```python
from build123d import *

# Parameters (mm, degrees)
SKETCH1_W           = 19.05
SKETCH1_H           = 22.225
BASE_FLANGE1_DEPTH  = 3.175
EDGE_FLANGE1_DEPTH  = 22.225
EDGE_FLANGE2_DEPTH  = 22.225
CUT_EXTRUDE1_DEPTH  = 42.119074421
SKETCH13_W          = 9.525
SKETCH13_H          = 3.175
BOSS_EXTRUDE1_DEPTH = 3.175
CUT_EXTRUDE2_DEPTH  = 35.761376285


# Sheet-metal steps are written as plain solids
with BuildPart() as part:
    # Sketch1 → Base-Flange1 (new body)
    with BuildSketch(Plane.XY):
        Rectangle(SKETCH1_W, SKETCH1_H)
    extrude(amount=-BASE_FLANGE1_DEPTH)

    # Edge-Flange1 section (across the edge) → Edge-Flange1 (add)
    with BuildSketch(Plane(origin=(10.525, 11.1125, -3.175), x_dir=(-1, 0, 0), z_dir=(0, -1, 0))):
        with BuildLine():
            Line((-3.175, 1), (-3.175, 25.4))
            Line((-3.175, 25.4), (0, 25.4))
            Line((0, 25.4), (0, 1))
            ThreePointArc((0, 1), (0.292893219, 0.292893219), (1, 0))
            Line((1, 0), (1, -3.175))
            ThreePointArc((1, -3.175), (-1.952170811, -1.952170811), (-3.175, 1))
        make_face()
    extrude(amount=EDGE_FLANGE1_DEPTH)

    # Edge-Flange2 section (across the edge) → Edge-Flange2 (add)
    with BuildSketch(Plane(origin=(-10.525, -11.1125, -3.175), x_dir=(1, 0, 0), z_dir=(0, 1, 0))):
        with BuildLine():
            Line((-3.175, 1), (-3.175, 25.4))
            Line((-3.175, 25.4), (0, 25.4))
            Line((0, 25.4), (0, 1))
            ThreePointArc((0, 1), (0.292893219, 0.292893219), (1, 0))
            Line((1, 0), (1, -3.175))
            ThreePointArc((1, -3.175), (-1.952170811, -1.952170811), (-3.175, 1))
        make_face()
    extrude(amount=EDGE_FLANGE2_DEPTH)

    # Sketch12 → Cut-Extrude1 (cut, through all)
    with BuildSketch(Plane(origin=(13.7, 0, 0), x_dir=(0, 0, -1), z_dir=(1, 0, 0))):
        Polygon((28.575, 11.1125), (7.35, 11.1125), (28.575, -7.9375), align=None)
    extrude(amount=-CUT_EXTRUDE1_DEPTH, mode=Mode.SUBTRACT)

    # Sketch13 → Boss-Extrude1 (add)
    with BuildSketch(Plane.XZ.offset(11.1125)):
        with Locations((0, -1.5875)):
            Rectangle(SKETCH13_W, SKETCH13_H)
    extrude(amount=BOSS_EXTRUDE1_DEPTH)

    # Sketch14 → Cut-Extrude2 (cut, through all)
    with BuildSketch(Plane.XY):
        with BuildLine():
            ThreePointArc((-3, 1.5875), (0, -1.4125), (3, 1.5875))
            Line((3, 1.5875), (-3, 1.5875))
        make_face()
        with BuildLine():
            Line((-3, 1.5875), (3, 1.5875))
            ThreePointArc((3, 1.5875), (0, 4.5875), (-3, 1.5875))
        make_face()
    extrude(amount=-CUT_EXTRUDE2_DEPTH, mode=Mode.SUBTRACT)


solid = part.part
```
Input: part model. Units: mm. Frame: model coordinates. A direction names the side the tool comes from. Give positions to 0.01 mm unless a question says otherwise; leave off trailing zeros. Loops run counter-clockwise (first coordinate to the right, second up) from the corner with the lowest first, then second, coordinate; pieces in that order, holes last. Notation, with made-up numbers: (42, -1.75) -> (56, -1.75) arc R35 cw to (56, 31.25) -> close; hole circle Ø2 at (-23.75, -24.5). An arc over 180 degrees is marked (long way). Use a Markdown table: item, result.
Q1. Section query B-B, the plane y = 1. Return the cut outline in (x, z) (3 decimals), plus the area to 3 significant figures.
Entries:
| item | result |
|---|---|
| outline | (-13.7, -18.617) -> (-10.525, -18.617) -> (-10.525, -4.175) arc R1 cw to (-9.525, -3.175) -> (-2.942, -3.175) -> (-2.942, 0) -> (-9.525, 0) arc R4.175 ccw to (-13.7, -4.175) -> close; (2.942, -3.175) -> (9.525, -3.175) arc R1 cw to (10.525, -4.175) -> (10.525, -18.617) -> (13.7, -18.617) -> (13.7, -4.175) arc R4.175 ccw to (9.525, 0) -> (2.942, 0) -> close |
| area | 159 mm² |
Q2. Section query D-D, the plane y = -8.5. Return the cut outline in (x, z) (3 decimals), plus the area to 3 significant figures.
Entries:
| item | result |
|---|---|
| outline | (-13.7, -28.575) -> (-10.525, -28.575) -> (-10.525, -4.175) arc R1 cw to (-9.525, -3.175) -> (9.525, -3.175) arc R1 cw to (10.525, -4.175) -> (10.525, -28.575) -> (13.7, -28.575) -> (13.7, -4.175) arc R4.175 ccw to (9.525, 0) -> (-9.525, 0) arc R4.175 ccw to (-13.7, -4.175) -> close |
| area | 241 mm² |
Q3. Access query for faces 1 (the flat face through (11, -11.112, -11)), 2 (the flat face through (-11, -11.112, -11)), 3 (the cylindrical face through (-10.24, -0.156, -3.476)). Directions: +Z, -Z, +X, -X, +Y, -Y. A direction counts if a zero-diameter tool reaches every point of the face in a straight line with its end or side. Return the directions, or none.
Entries:
| item | result |
|---|---|
| face 1 | +Z, -Z, +X, -Y |
| face 2 | +Z, -Z, -X, -Y |
| face 3 | -Z, +Y, -Y |
Q4. Ray query, probe 1 along Y at (x, z) = (0, -2.5); probe 2 along X at (y, z) = (-10.75, -7.25) (3 decimals); probe 3 along Y at (x, z) = (12.75, -8). Return the intervals inside material, ascending. Write a range as from..to.
Entries:
| item | result |
|---|---|
| probe 1 | y = -14.29..-1.41, 4.59..11.11 |
| probe 2 | x = -13.7..-10.525, 10.525..13.7 |
| probe 3 | y = -11.11..10.53 |
Q5. Pull-direction query (X, two-part tool) for faces 4 (the flat face through (0, 11.112, -3)), 5 (the cylindrical face through (10.24, 0.156, -3.476)), 6 (the flat face through (10.525, -2, -14)), 7 (the flat face through (-4.762, -13, -2)); classes: pulls with the +X half, pulls with the -X half, needs draft (parallel to the pull), parting line crosses it, or undercut.
Entries:
| item | result |
|---|---|
| face 4 | needs draft |
| face 5 | undercut |
| face 6 | undercut |
| face 7 | pulls with the -X half |
Q6. First-contact query: P1, Ø1.6, axis at y = -12, z = -1.5, coming from the -X side; P2, Ø8, axis at x = 5, y = 4, coming from the -Z side (3 decimals); P3, Ø3.5, axis at x = 0, y = 1.59, coming from the -Z side; P4, Ø10, axis at x = -10, z = -19, coming from the -Y side. Flat tips, straight axial feed; report the tip coordinate or a pass-through.
Entries:
| item | result |
|---|---|
| P1 | stops at x = -4.76 |
| P2 | stops at z = -3.175 |
| P3 | passes through |
| P4 | stops at y = -11.11 |
Q7. Section query C-C, the plane z = -11.75. Return the cut outline in (x, y) (1 decimal).
Entries:
| item | result |
|---|---|
| outline | (-13.7, -11.1) -> (-10.5, -11.1) -> (-10.5, 7.2) -> (-13.7, 7.2) -> close; (10.5, -11.1) -> (13.7, -11.1) -> (13.7, 7.2) -> (10.5, 7.2) -> close |
Q8. Section query A-A, the plane x = 0. Return the cut outline in (y, z) (1 decimal).
Entries:
| item | result |
|---|---|
| outline | (-14.3, -3.2) -> (-1.4, -3.2) -> (-1.4, 0) -> (-14.3, 0) -> close; (4.6, -3.2) -> (11.1, -3.2) -> (11.1, 0) -> (4.6, 0) -> close |
